CAD build for the part. Positions are in the model's coordinates, mm. Give positions to 0.01 mm unless a question says otherwise; leave off trailing zeros. Write each loop counter-clockwise with the first axis right and the second up, starting at its lowest first coordinate (ties: lowest second). Pieces come first, ordered by that corner, then holes. Notation, with made-up numbers: (63, 17.25) -> (75, 17.25) arc R16 cw to (75, 31.25) -> close; hole circle Ø5 at (36.25, 4.25). An arc over 180 degrees is marked (long way). Answer as a JSON object with one key per item and string values.
```python
from build123d import *

# Parameters (mm, degrees)
SKETCH1_R           = 2
BOSS_EXTRUDE1_DEPTH = 2
SKETCH2_R           = 2.5
CUT_EXTRUDE1_DEPTH  = 2


with BuildPart() as part:
    # Sketch1 → Boss-Extrude1 (new body)
    with BuildSketch(Plane(origin=(0, 0, 0), x_dir=(1, 0, 0), z_dir=(0, 1, 0))):
        with BuildLine():
            Line((-5.656854249, 0), (-20.329319959, -14.67246571))
            ThreePointArc((-20.329319959, -14.67246571), (-20.329319959, -20.329319959), (-14.67246571, -20.329319959))
            Line((-14.67246571, -20.329319959), (0, -5.656854249))
            Line((0, -5.656854249), (14.67246571, -20.329319959))
            ThreePointArc((14.67246571, -20.329319959), (20.329319959, -20.329319959), (20.329319959, -14.67246571))
            Line((20.329319959, -14.67246571), (5.656854249, 0))
            Line((5.656854249, 0), (20.329319959, 14.67246571))
            ThreePointArc((20.329319959, 14.67246571), (20.329319959, 20.329319959), (14.67246571, 20.329319959))
            Line((14.67246571, 20.329319959), (0, 5.656854249))
            Line((0, 5.656854249), (-14.67246571, 20.329319959))
            ThreePointArc((-14.67246571, 20.329319959), (-20.329319959, 20.329319959), (-20.329319959, 14.67246571))
            Line((-20.329319959, 14.67246571), (-5.656854249, 0))
        make_face()
        with Locations((-17.500892834, 17.500892834)):
            Circle(SKETCH1_R, mode=Mode.SUBTRACT)
        with Locations((17.500892834, 17.500892834)):
            Circle(SKETCH1_R, mode=Mode.SUBTRACT)
        with Locations((17.500892834, -17.500892834)):
            Circle(SKETCH1_R, mode=Mode.SUBTRACT)
        with Locations((-17.500892834, -17.500892834)):
            Circle(SKETCH1_R, mode=Mode.SUBTRACT)
    extrude(amount=BOSS_EXTRUDE1_DEPTH)

    # Sketch2 → Cut-Extrude1 (cut)
    with BuildSketch(Plane(origin=(0, 2, 0), x_dir=(1, 0, 0), z_dir=(0, 1, 0))):
        Circle(SKETCH2_R)
    extrude(amount=-CUT_EXTRUDE1_DEPTH, mode=Mode.SUBTRACT)


solid = part.part
```
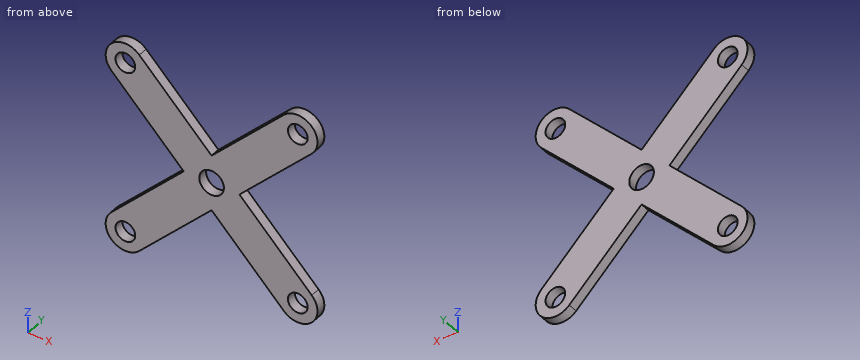
1) Slice it at A-A (x = 18.5). List the corners of the cut face in (y, z), then the cut area to 3 significant figures.
Model answer:
{"outline": "(0, -21.37) -> (2, -21.37) -> (2, -19.23) -> (0, -19.23) -> close; (0, -15.77) -> (2, -15.77) -> (2, -12.84) -> (0, -12.84) -> close; (0, 12.84) -> (2, 12.84) -> (2, 15.77) -> (0, 15.77) -> close; (0, 19.23) -> (2, 19.23) -> (2, 21.37) -> (0, 21.37) -> close", "area": "20.3 mm2"}
2) Slice it at D-D (x = 9). List the corners of the cut face in (y, z), then the cut area to 3 significant figures.
Model answer:
{"outline": "(0, -14.66) -> (2, -14.66) -> (2, -3.34) -> (0, -3.34) -> close; (0, 3.34) -> (2, 3.34) -> (2, 14.66) -> (0, 14.66) -> close", "area": "45.3 mm2"}
3) Pin check, flat tip, straight feed: pin 1 (4 mm diameter, centred on x = 0, z = 0, fed in from -Y). Stop position of the tip, or through.
Model answer:
{"pin 1": "passes through"}
4) Slice it at B-B (z = -1.5). List the corners of the cut face in (x, y).
Model answer:
{"outline": "(-7.16, 0) -> (-2, 0) -> (-2, 2) -> (-7.16, 2) -> close; (2, 0) -> (7.16, 0) -> (7.16, 2) -> (2, 2) -> close"}
5) Slice it at C-C (y = 0.95). List the corners of the cut face in (x, z).
Model answer:
{"outline": "(-20.33, -14.67) arc R4 ccw to (-14.67, -20.33) -> (0, -5.66) -> (14.67, -20.33) arc R4 ccw to (20.33, -14.67) -> (5.66, 0) -> (20.33, 14.67) arc R4 ccw to (14.67, 20.33) -> (0, 5.66) -> (-14.67, 20.33) arc R4 ccw to (-20.33, 14.67) -> (-5.66, 0) -> close; hole circle Ø4 at (-17.5, -17.5); hole circle Ø4 at (-17.5, 17.5); hole circle Ø5 at (0, 0); hole circle Ø4 at (17.5, -17.5); hole circle Ø4 at (17.5, 17.5)"}
6) Wall check: probe 1 along Z at (x, y) = (-18.5, 1.15); probe 2 along Z at (x, y) = (-8.5, 1.8); probe 3 along X at (y, z) = (1.25, -19). Give the ranges that are in metal, low to high.
Model answer:
{"probe 1": "z = -21.37 to -19.23, -15.77 to -12.84, 12.84 to 15.77, 19.23 to 21.37", "probe 2": "z = -14.16 to -2.84, 2.84 to 14.16", "probe 3": "x = -21.21 to -18.82, -16.18 to -13.34, 13.34 to 16.18, 18.82 to 21.21"}
